Model file for the job. Use its own axes, mm. A direction names the side the tool comes from. Give positions to 0.01 mm unless a question says otherwise; leave off trailing zeros. Loops run counter-clockwise (first coordinate to the right, second up) from the corner with the lowest first, then second, coordinate; pieces in that order, holes last. Notation, with made-up numbers: M -8.75,-36.5 L 45.25,-36.5 A23 cw 45.25,2.5 Z; hole C 40,54 d9. An arc over 180 degrees is marked long. Answer in a Markdown table with one row per item.
```python
from build123d import *

# Parameters (mm, degrees)
BOSS_EXTRUDE1_DEPTH      = 500
BOSS_EXTRUDE1_DEPTH_BACK = 1600
SKETCH1_W                = 150
SKETCH1_H                = 300
CUT_EXTRUDE1_DEPTH       = 2309
SKETCH5_W                = 150
SKETCH5_H                = 300
BOSS_EXTRUDE2_DEPTH      = 350
SKETCH6_W                = 210
SKETCH6_H                = 250
CUT_EXTRUDE4_DEPTH       = 45
CUT_EXTRUDE5_DEPTH       = 1500
CUT_EXTRUDE7_DEPTH       = 355
FILLET8_R                = 1.5
FILLET9_R                = 1.5
SKETCH9_W                = 150
SKETCH9_H                = 300
BOSS_EXTRUDE3_DEPTH      = 300
SKETCH10_W               = 70
SKETCH10_H               = 230
CUT_EXTRUDE17_DEPTH      = 140
SKETCH11_W               = 125
SKETCH11_H               = 10.75
BOSS_EXTRUDE4_DEPTH      = 300
CUT_EXTRUDE18_DEPTH      = 394
SWEEP1_PROFILE_R         = 7.5
SKETCH50_R               = 4.335134875
BOSS_EXTRUDE5_DEPTH      = 20
CUT_EXTRUDE19_DEPTH      = 30
CUT_EXTRUDE19_DEPTH_BACK = 250
SKETCH82_W               = 45
SKETCH82_H               = 30
CUT_EXTRUDE20_DEPTH      = 32
CUT_EXTRUDE20_DEPTH_BACK = 250
SKETCH85_W               = 45
SKETCH85_H               = 30


with BuildPart() as part:
    # Sketch1 → Boss-Extrude1 (new, two sides: drawn at the far end of the back side and taken through both)
    with BuildSketch(Plane.XY.offset(-BOSS_EXTRUDE1_DEPTH_BACK)):
        with Locations((375, -2.824081205)):
            Rectangle(SKETCH1_W, SKETCH1_H)
    extrude(amount=BOSS_EXTRUDE1_DEPTH + BOSS_EXTRUDE1_DEPTH_BACK)

    # Sketch2 → Cut-Extrude1 (cut)
    with BuildSketch(Plane(origin=(0, 0, -1600), x_dir=(-1, 0, 0), z_dir=(0, 0, -1))):
        Polygon((-300, 49.675918795), (-300, 69.675918795), (-325, 69.675918795), (-325, 77.175918795), (-345, 77.175918795), (-345, 42.175918795), (-325, 42.175918795), (-325, 49.675918795), align=None)
        Polygon((-300, 129.675918795), (-325, 129.675918795), (-325, 137.175918795), (-345, 137.175918795), (-345, 102.175918795), (-325, 102.175918795), (-325, 109.675918795), (-300, 109.675918795), align=None)
        Polygon((-300, -10.324081205), (-300, 9.675918795), (-325, 9.675918795), (-325, 17.175918795), (-345, 17.175918795), (-345, -17.824081205), (-325, -17.824081205), (-325, -10.324081205), align=None)
        Polygon((-300, -70.324081205), (-300, -50.324081205), (-325, -50.324081205), (-325, -42.824081205), (-345, -42.824081205), (-345, -77.824081205), (-325, -77.824081205), (-325, -70.324081205), align=None)
        Polygon((-300, -130.324081205), (-300, -110.324081205), (-325, -110.324081205), (-325, -102.824081205), (-345, -102.824081205), (-345, -137.824081205), (-325, -137.824081205), (-325, -130.324081205), align=None)
    extrude(amount=-CUT_EXTRUDE1_DEPTH, mode=Mode.SUBTRACT)

    # Sketch5 → Boss-Extrude2 (add)
    with BuildSketch(Plane.XY.offset(500)):
        with Locations((375, -2.824081205)):
            Rectangle(SKETCH5_W, SKETCH5_H)
    extrude(amount=BOSS_EXTRUDE2_DEPTH)

    # Sketch6 → Cut-Extrude4 (cut)
    with BuildSketch(Plane.ZY.offset(-300)):
        with Locations((685, -2.824081205)):
            Rectangle(SKETCH6_W, SKETCH6_H)
    extrude(amount=-CUT_EXTRUDE4_DEPTH, mode=Mode.SUBTRACT)

    # Sketch7 → Cut-Extrude5 (cut, symmetric)
    with BuildSketch(Plane.XZ.offset(-122.175918795)):
        Polygon((300, 580), (345, 790), (300, 790), align=None)
    extrude(amount=CUT_EXTRUDE5_DEPTH, both=True, mode=Mode.SUBTRACT)

    # Sketch8 → Cut-Extrude7 (cut)
    with BuildSketch(Plane.XZ.offset(152.824081205)):
        Polygon((450, 850), (450, 800.747642435), (325, 800.747642435), (325, 790), (300, 790), (300, 850), align=None)
    extrude(amount=-CUT_EXTRUDE7_DEPTH, mode=Mode.SUBTRACT)

    # Fillet8
    fillet8_edges = [part.edges().sort_by_distance(p)[0] for p in [
        (325, -2.824081205, 790),
        (325, 147.175918795, 795.373821218),
        (325, -2.824081205, 800.747642435),
        (325, -152.824081205, 795.373821218),
    ]]
    fillet(fillet8_edges, radius=FILLET8_R)

    # Fillet9
    fillet9_edges = [part.edges().sort_by_distance(p)[0] for p in [
        (322.5, -152.824081205, 685),
        (322.5, 147.175918795, 685),
        (322.5, 122.175918795, 685),
        (322.5, -127.824081205, 685),
    ]]
    fillet(fillet9_edges, radius=FILLET9_R)

    # Sketch9 → Boss-Extrude3 (add)
    with BuildSketch(Plane(origin=(0, 0, -1600), x_dir=(-1, 0, 0), z_dir=(0, 0, -1))):
        with Locations((-375, -2.824081205)):
            Rectangle(SKETCH9_W, SKETCH9_H)
    extrude(amount=BOSS_EXTRUDE3_DEPTH)

    # Sketch10 → Cut-Extrude17 (cut, symmetric)
    with BuildSketch(Plane(origin=(0, -2.824081205, 0), x_dir=(-1, 0, 0), z_dir=(0, -1, 0))):
        with Locations((-335, 1785)):
            Rectangle(SKETCH10_W, SKETCH10_H)
    extrude(amount=CUT_EXTRUDE17_DEPTH, both=True, mode=Mode.SUBTRACT)

    # Sketch11 → Boss-Extrude4 (add)
    with BuildSketch(Plane.XZ.offset(152.824081205)):
        with Locations((387.5, -1905.375)):
            Rectangle(SKETCH11_W, SKETCH11_H)
    extrude(amount=-BOSS_EXTRUDE4_DEPTH)

    # Sketch13 → Cut-Extrude18 (cut)
    with BuildSketch(Plane.XZ.offset(152.824081205)):
        Polygon((300, -1900), (345.980080602, -1900), (300, -1670), align=None)
    extrude(amount=-CUT_EXTRUDE18_DEPTH, mode=Mode.SUBTRACT)

    # Sweep1: sweep along a path in Sketch15
    with BuildLine(Plane.XY.offset(-1449.252357565)) as sweep1_path:
        Line((350, -145.902648046), (350, -197.264838167))
        ThreePointArc((350, -197.264838167), (347.071067812, -204.335905979), (340, -207.264838167))
        Line((340, -207.264838167), (304.112930958, -207.264838167))
    # Sweep1 profile (on start of the path) → Sweep1 (sweep)
    with BuildSketch(Plane(origin=(350, -145.902648046, -1449.252357565), x_dir=(0, 0, -1), z_dir=(0, -1, 0))):
        Circle(SWEEP1_PROFILE_R)
    sweep(path=sweep1_path.line)

    # Sketch50 → Boss-Extrude5 (add)
    with BuildSketch(Plane.ZY.offset(-304.112930958)):
        with Locations((-1449.252357565, -207.264838167)):
            Circle(SKETCH50_R)
    extrude(amount=BOSS_EXTRUDE5_DEPTH)

    # Sketch82 → Cut-Extrude19 (cut, two sides: drawn at the far end of the back side and taken through both)
    with BuildSketch(Plane.XZ.offset(110.324081205).offset(-CUT_EXTRUDE19_DEPTH_BACK)):
        with Locations((322.5, -1545)):
            Rectangle(SKETCH82_W, SKETCH82_H)
    extrude(amount=CUT_EXTRUDE19_DEPTH + CUT_EXTRUDE19_DEPTH_BACK, mode=Mode.SUBTRACT)

    # Sketch85 → Cut-Extrude20 (cut, two sides: drawn at the far end of the back side and taken through both)
    with BuildSketch(Plane.XZ.offset(110.324081205).offset(-CUT_EXTRUDE20_DEPTH_BACK)):
        with Locations((322.5, 445)):
            Rectangle(SKETCH85_W, SKETCH85_H)
    extrude(amount=CUT_EXTRUDE20_DEPTH + CUT_EXTRUDE20_DEPTH_BACK, mode=Mode.SUBTRACT)


solid = part.part
```
Q1. Saw through at A-A (x = 425.5). Give the cut face in (y, z), and give its area (3 significant figures).
Reported:
| item | result |
|---|---|
| outline | M -152.82,-1910.75 L 147.18,-1910.75 L 147.18,800.75 L -152.82,800.75 Z |
| area | 813,000 mm² |
Q2. Probe probe 1 along Y at (x, z) = (307, -1467); probe 2 along Y at (x, z) = (338, -1578); probe 3 along Z at (x, y) = (317, -34.5). List the from-to ranges inside material, lowest first.
Reported:
| item | result |
|---|---|
| probe 1 | -152.82 to -130.32, -110.32 to -70.32, -50.32 to -10.32, 9.68 to 49.68, 69.68 to 109.68, 129.68 to 147.18 |
| probe 2 | -152.82 to -137.82, -102.82 to -77.82, -42.82 to -17.82, 17.18 to 42.18, 77.18 to 102.18, 137.18 to 147.18 |
| probe 3 | -1670 to -1560, -1530 to 430, 460 to 580 |
Q3. Drop flat-ended pins along their axis: pin 1 (10.5 mm diameter, centred on x = 319, y = -120.5, fed in from -Z); pin 2 (4 mm diameter, centred on x = 412, z = 62, fed in from -Y); pin 3 (8 mm diameter, centred on y = -34, z = -1112, fed in from -X). Give the stop position or say it passes through.
Reported:
| item | result |
|---|---|
| pin 1 | z = -1670 |
| pin 2 | y = -152.82 |
| pin 3 | x = 300 |
Q4. 3-axis set-ups, long thin cutter, end or side, ignore diameter. For faces 1 (the face through (335, -5, -1670)), 2 (the face through (323.31, -147.89, -1786.61)), 3 (the face through (321.92, -152.4, 680.12)), 4 (the face through (321.92, 146.75, 680.12)), 5 (the face through (374, 147.176, -536)): which of +Z, -Z, +X, -X, +Y, -Y reach the whole face in a straight line?
Reported:
| item | result |
|---|---|
| face 1 | -X |
| face 2 | -X, +Y, -Y |
| face 3 | -X, -Y |
| face 4 | -X, +Y |
| face 5 | +Z, -Z, +X, -X, +Y |
